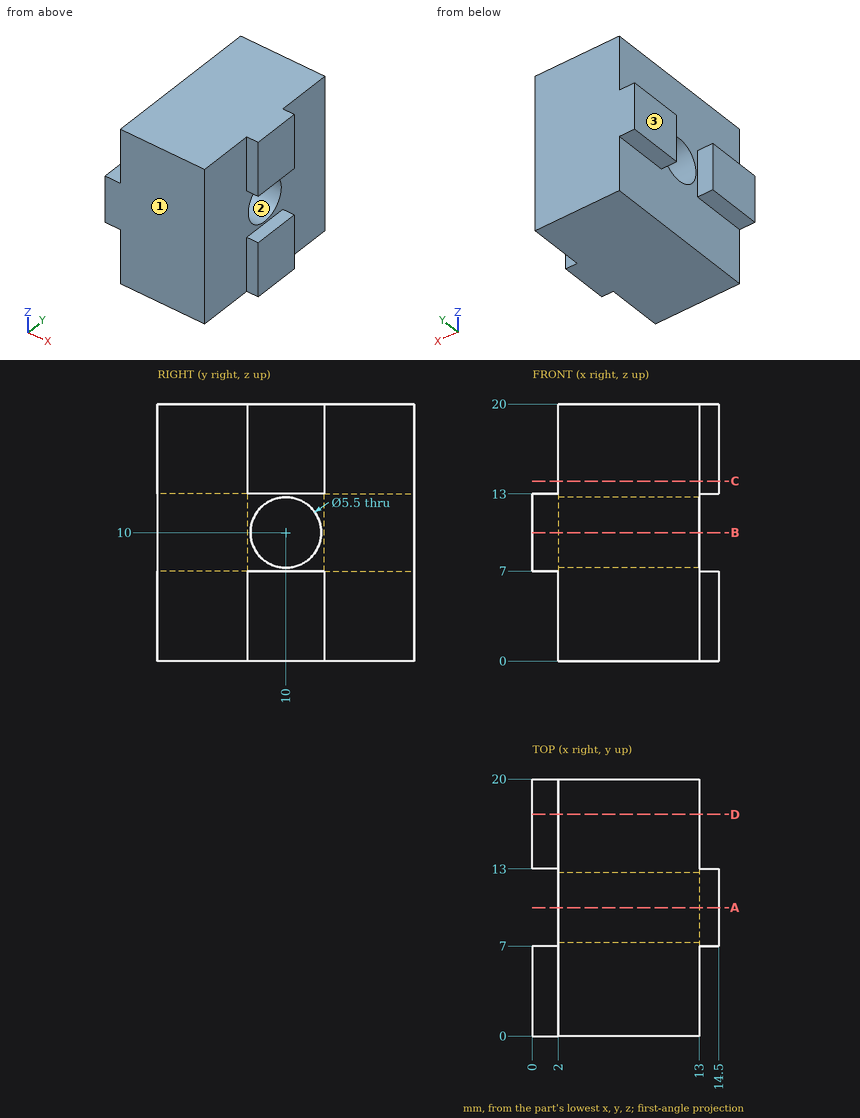
Geometry check sheet. Reference: drawing and pictorial views, mm from the part's lowest x, y, z. Coordinates: 2 decimals unless noted, no trailing zeros. Write each loop counter-clockwise with the first axis right and the second up, starting at its lowest first coordinate (ties: lowest second). Pieces come first, ordered by that corner, then holes. Notation, with made-up numbers: M 80,88 L 106,88 A7 cw 106,93 Z; hole C 36.5,51 d8. An arc over 180 degrees is marked long. Use one line per item in the form item = value.
Item 1: Sectioned sample at D-D, the plane y = 17.25. Record the cut outline in (x, z).
Answer below:
outline = M 0,7 L 2,7 L 2,0 L 13,0 L 13,20 L 2,20 L 2,13 L 0,13 Z
Item 2: Sectioned sample at B-B, the plane z = 10. Record the cut outline in (x, y), and give its area (4 significant figures).
Answer below:
outline = M 0,0 L 13,0 L 13,7.25 L 2,7.25 L 2,7 L 0,7 Z; M 0,13 L 2,13 L 2,12.75 L 13,12.75 L 13,20 L 0,20 Z
area = 187.5 mm^2
Item 3: Sectioned sample at C-C, the plane z = 14. Record the cut outline in (x, y).
Answer below:
outline = M 2,0 L 13,0 L 13,7 L 14.5,7 L 14.5,13 L 13,13 L 13,20 L 2,20 Z
Item 4: Material ranges on L1, parallel to Z at x = 9.5, y = 10; L2, parallel to X at y = 6, z = 16, recorded low to high. Write a range as from..to.
Answer below:
L1 = 0..7.25, 12.75..20
L2 = 2..13
Item 5: Release check for a two-part mould opening along Y. For the marked faces 1, 2 and 3 record: pulls with the +Y half, pulls with the -Y half, needs draft (parallel to the pull), parting line crosses it, or undercut.
Answer below:
face_1 = pulls with the -Y half
face_2 = undercut
face_3 = needs draft
Item 6: Gauge pin test, flat ends, axial feed: pin 1 Ø7 at (y, z) = (10, 10) entering from +X; pin 2 Ø1 at (x, y) = (1, 5) entering from +Z; pin 3 Ø0.8 at (x, z) = (13.5, 4.5) entering from +Y; pin 4 Ø1 at (y, z) = (5.5, 11.5) entering from +X. Record the tip position at first contact, or that the pin passes through.
Answer below:
pin_1 = 14.5
pin_2 = 13
pin_3 = 13
pin_4 = 13
Item 7: Sectioned sample at A-A, the plane y = 10. Record the cut outline in (x, z), and give its area (4 significant figures).
Answer below:
outline = M 2,0 L 14.5,0 L 14.5,7 L 13,7 L 13,7.25 L 2,7.25 Z; M 2,12.75 L 13,12.75 L 13,13 L 14.5,13 L 14.5,20 L 2,20 Z
area = 180.5 mm^2
